Read the model definition and answer for the solid it produces. Units are mm, in the model's axes. A direction names the side the tool comes from. Give positions to 0.01 mm unless a question says otherwise; leave off trailing zeros. Order: outer loops, then holes, each group sorted by start corner. A loop starts at its lowest first (then second) coordinate and runs counter-clockwise, first axis right, second up. Notation, with made-up numbers: (2.25, -11) -> (34.25, -11) arc R18 ccw to (34.25, 6) -> close; hole circle Ø4 at (27.5, 17.25). An arc over 180 degrees is marked (long way). Use one line per item in the form item = value.
```python
from build123d import *

# Parameters (mm, degrees)
SKETCH1_W               = 40
SKETCH1_H               = 9
BOSS_EXTRUDE1_DEPTH     = 5
SKETCH2_W               = 40
SKETCH2_H               = 3
BOSS_EXTRUDE4_DEPTH     = 10
CUT_EXTRUDE5_DEPTH      = 26.401771592
CUT_EXTRUDE5_DEPTH_BACK = 12.5
SKETCH4_R               = 2.75
CUT_EXTRUDE6_DEPTH      = 25.010414407
CUT_EXTRUDE6_DEPTH_BACK = 25.010414407
SKETCH5_R               = 1.5
CUT_EXTRUDE7_DEPTH      = 27.570660511
CUT_EXTRUDE7_DEPTH_BACK = 27.570660511
SKETCH6_R               = 1.5


with BuildPart() as part:
    # Sketch1 → Boss-Extrude1 (new body)
    with BuildSketch(Plane(origin=(0, 0, 0), x_dir=(1, 0, 0), z_dir=(0, 1, 0))):
        Rectangle(SKETCH1_W, SKETCH1_H)
    extrude(amount=BOSS_EXTRUDE1_DEPTH)

    # Sketch2 → Boss-Extrude4 (add)
    with BuildSketch(Plane(origin=(0, 5, 0), x_dir=(1, 0, 0), z_dir=(0, 1, 0))):
        with Locations((0, 3)):
            Rectangle(SKETCH2_W, SKETCH2_H)
        with Locations((0, -3)):
            Rectangle(SKETCH2_W, SKETCH2_H)
    extrude(amount=BOSS_EXTRUDE4_DEPTH)

    # Sketch4 → Cut-Extrude5 (cut, two sides: drawn at the far end of the back side and taken through both)
    with BuildSketch(Plane(origin=(0, 15, 0), x_dir=(1, 0, 0), z_dir=(0, 1, 0)).offset(-CUT_EXTRUDE5_DEPTH_BACK)):
        with Locations(Location((-10, 0, 0), (0, 0, 146.944268849))):
            Circle(SKETCH4_R)
        with Locations(Location((10, 0, 0), (0, 0, 90))):
            Circle(SKETCH4_R)
    extrude(amount=CUT_EXTRUDE5_DEPTH + CUT_EXTRUDE5_DEPTH_BACK, mode=Mode.SUBTRACT)

    # Sketch5 → Cut-Extrude6 (cut, two sides: drawn at the far end of the back side and taken through both)
    with BuildSketch(Plane(origin=(0, 2.5, 0), x_dir=(1, 0, 0), z_dir=(0, 1, 0)).offset(-CUT_EXTRUDE6_DEPTH_BACK)):
        with Locations(Location((-10, 0, 0), (0, 0, 270))):
            Circle(SKETCH5_R)
        with Locations(Location((10, 0, 0), (0, 0, 270))):
            Circle(SKETCH5_R)
    extrude(amount=CUT_EXTRUDE6_DEPTH + CUT_EXTRUDE6_DEPTH_BACK, mode=Mode.SUBTRACT)

    # Sketch6 → Cut-Extrude7 (cut, two sides: drawn at the far end of the back side and taken through both)
    with BuildSketch(Plane.XY.offset(4.5).offset(-CUT_EXTRUDE7_DEPTH_BACK)):
        with Locations((-10, 10)):
            Circle(SKETCH6_R)
        with Locations((10, 10)):
            Circle(SKETCH6_R)
    extrude(amount=CUT_EXTRUDE7_DEPTH + CUT_EXTRUDE7_DEPTH_BACK, mode=Mode.SUBTRACT)


solid = part.part
```
Item 1: The part is cut by section A-A on y = 10. State how many separate pieces and enclosed holes the cut face has, and give its area (3 significant figures).
Checks:
separate_pieces = 6
enclosed_holes = 0
area = 201 mm²
Item 2: Determine the mould class of faces 1 (the cylindrical face through (-8.614, 9.425, -3.418)), 2 (the flat face through (0, 7, -4.5)), 3 (the cylindrical face through (11.386, 9.425, -3.418)), 4 (the flat face through (-10, 2.5, -2)) for opening direction Y: +Y half, -Y half, draft (parallel to the pull), parting line (faces both ways), or undercut.
Checks:
face_1 = undercut
face_2 = draft
face_3 = undercut
face_4 = +Y half
Item 3: The part is cut by section C-C on z = 0. Give the vertices of the cut face in (x, y), and give its area (4 significant figures).
Checks:
outline = (-20, 0) -> (-11.5, 0) -> (-11.5, 2.5) -> (-12.75, 2.5) -> (-12.75, 5) -> (-20, 5) -> close; (-8.5, 0) -> (8.5, 0) -> (8.5, 2.5) -> (7.25, 2.5) -> (7.25, 5) -> (-7.25, 5) -> (-7.25, 2.5) -> (-8.5, 2.5) -> close; (11.5, 0) -> (20, 0) -> (20, 5) -> (12.75, 5) -> (12.75, 2.5) -> (11.5, 2.5) -> close
area = 157.5 mm²
Item 4: Straight lines are drawn through the part: L1, parallel to X at y = 3.75, z = 1.75; L2, parallel to X at y = 4.75, z = -2.5; L3, parallel to Z at x = -2, y = 14. For each, find the intervals that lie inside material, in ascending order. Write a range as from..to.
Checks:
L1 = -20..-12.12, -7.88..7.88, 12.12..20
L2 = -20..-11.15, -8.85..8.85, 11.15..20
L3 = -4.5..-1.5, 1.5..4.5
Item 5: The part is cut by section B-B on x = -10. Give the vertices of the cut face in (y, z).
Checks:
outline = (0, -4.5) -> (8.5, -4.5) -> (8.5, -2.75) -> (2.5, -2.75) -> (2.5, -1.5) -> (0, -1.5) -> close; (0, 1.5) -> (2.5, 1.5) -> (2.5, 2.75) -> (8.5, 2.75) -> (8.5, 4.5) -> (0, 4.5) -> close; (11.5, -4.5) -> (15, -4.5) -> (15, -2.75) -> (11.5, -2.75) -> close; (11.5, 2.75) -> (15, 2.75) -> (15, 4.5) -> (11.5, 4.5) -> close
Item 6: Given pin 1 Ø1.6 at (x, z) = (10.5, 0) entering from +Y; pin 2 Ø1.5 at (x, z) = (-0.5, 0.5) entering from +Y, each flat-ended and moving along its own axis, determine where each tip first touches the part or whether it passes through.
Checks:
pin_1 = through
pin_2 = 5
Item 7: The part is cut by section D-D on x = -1. Give the vertices of the cut face in (y, z), and give its area (3 significant figures).
Checks:
outline = (0, -4.5) -> (15, -4.5) -> (15, -1.5) -> (5, -1.5) -> (5, 1.5) -> (15, 1.5) -> (15, 4.5) -> (0, 4.5) -> close
area = 105 mm²
Item 8: Which of the six approach directions +Z, -Z, +X, -X, +Y, -Y give full straight-line access (tool end or side, diameter ignored) to faces 5 (the cylindrical face through (9.879, 7.274, 2.747)), 6 (the flat face through (0, 10, 1.5)), 7 (the flat face through (20, 7, 2))?
Checks:
face_5 = +Y
face_6 = +X, -X, +Y
face_7 = +Z, -Z, +X, +Y, -Y
